Work out the finished part from the listing and answer in its coordinate system (mm). A direction names the side the tool comes from. Coordinates: 2 decimals unless noted, no trailing zeros. Order: outer loops, then holes, each group sorted by start corner. A loop starts at its lowest first (then second) coordinate and runs counter-clockwise, first axis right, second up.
1. The part is cut by section A-A, the plane y = 6. Give the vertices of the cut face in (x, z).
2. The part is cut by section B-B, the plane z = 0. Give the vertices of the cut face in (x, y).
3. Flat-ended cylindrical pins translate along their axes: pin 1 Ø1.2 at (y, z) = (2, -1.5) entering from +X; pin 2 Ø1.2 at (y, z) = (4.5, -2) entering from -X; pin 3 Ø1.2 at (x, y) = (5.5, 5) entering from +Z. Find the tip coordinate at first contact, or state that the pin passes through.
4. The part is cut by section D-D, the plane x = -3.75. Give the vertices of the cut face in (y, z).
5. Find the intervals of material crossed by probe 1 along Z at (x, y) = (-4.02, 7.4); probe 2 along Z at (x, y) = (3, 7.75); probe 3 along X at (y, z) = (4.25, 1.25), in increasing order.
6. Determine the mould class of faces 4 (the flat face through (0, 4, 3.65)), 5 (the flat face through (4.92, 4, 2)), 6 (the cylindrical face through (7.67, 3.85, -0.08)) for opening direction X: +X half, -X half, draft (parallel to the pull), parting line (faces both ways), or undercut.
7. A tool of negligible diameter and unlimited length cuts with its end or side. For faces 1 (the cylindrical face through (-7.067, 7.406, -0.134)), 2 (the flat face through (2, 4, 0.9)), 3 (the cylindrical face through (-7.067, 0.394, 0.134)), from which of +Z, -Z, +X, -X, +Y, -Y can it reach the whole face along a straight path? Write none if from no direction.
8. The part is cut by section C-C, the plane x = 4.5. Give the vertices of the cut face in (y, z), then the cut area to 3 significant figures.
```python
from build123d import *

# Parameters (mm, degrees)
SKETCH1_R           = 2.4
BOSS_EXTRUDE1_DEPTH = 7.8
SKETCH2_R           = 3.05
CUT_EXTRUDE1_DEPTH  = 0.8
SKETCH4_R           = 3.05
CUT_EXTRUDE2_DEPTH  = 0.8


with BuildPart() as part:
    # Sketch1 → Boss-Extrude1 (new body)
    with BuildSketch(Plane(origin=(0, 0, 0), x_dir=(1, 0, 0), z_dir=(0, 1, 0))):
        with BuildLine():
            Line((-4.02, 3.65), (4.02, 3.65))
            ThreePointArc((4.02, 3.65), (7.67, 0), (4.02, -3.65))
            Line((4.02, -3.65), (-4.02, -3.65))
            ThreePointArc((-4.02, -3.65), (-7.67, 0), (-4.02, 3.65))
        make_face()
        with Locations((-4.02, 0)):
            Circle(SKETCH1_R, mode=Mode.SUBTRACT)
        Polygon((3.12, 2.4), (3.12, 0.9), (1.62, 0.9), (1.62, -0.9), (3.12, -0.9), (3.12, -2.4), (4.92, -2.4), (4.92, -0.9), (6.42, -0.9), (6.42, 0.9), (4.92, 0.9), (4.92, 2.4), align=None, mode=Mode.SUBTRACT)
    extrude(amount=BOSS_EXTRUDE1_DEPTH)

    # Sketch2 → Cut-Extrude1 (cut)
    with BuildSketch(Plane(origin=(0, 7.8, 0), x_dir=(1, 0, 0), z_dir=(0, 1, 0))):
        with Locations((-4.02, 0)):
            Circle(SKETCH2_R)
    extrude(amount=-CUT_EXTRUDE1_DEPTH, mode=Mode.SUBTRACT)

    # Sketch4 → Cut-Extrude2 (cut)
    with BuildSketch(Plane.XZ):
        with Locations((-4.02, 0)):
            Circle(SKETCH4_R)
    extrude(amount=-CUT_EXTRUDE2_DEPTH, mode=Mode.SUBTRACT)


solid = part.part
```
Geometry says:
1. outline: (-4.02, -3.65) - (4.02, -3.65) arc R3.65 ccw to (4.02, 3.65) - (-4.02, 3.65) arc R3.65 ccw to start; hole circle Ø4.8 at (-4.02, 0); hole (1.62, -0.9) - (3.12, -0.9) - (3.12, -2.4) - (4.92, -2.4) - (4.92, -0.9) - (6.42, -0.9) - (6.42, 0.9) - (4.92, 0.9) - (4.92, 2.4) - (3.12, 2.4) - (3.12, 0.9) - (1.62, 0.9) - close
2. outline: (-7.67, 0) - (-7.07, 0) - (-7.07, 0.8) - (-6.42, 0.8) - (-6.42, 7) - (-7.07, 7) - (-7.07, 7.8) - (-7.67, 7.8) - close; (-1.62, 0.8) - (-0.97, 0.8) - (-0.97, 0) - (1.62, 0) - (1.62, 7.8) - (-0.97, 7.8) - (-0.97, 7) - (-1.62, 7) - close; (6.42, 0) - (7.67, 0) - (7.67, 7.8) - (6.42, 7.8) - close
3. pin 1: stops at x = 7.56
3. pin 2: stops at x = -7.39
3. pin 3: stops at z = 3.54
4. outline: (0, -3.65) - (7.8, -3.65) - (7.8, -3.04) - (7, -3.04) - (7, -2.38) - (0.8, -2.38) - (0.8, -3.04) - (0, -3.04) - close; (0, 3.04) - (0.8, 3.04) - (0.8, 2.38) - (7, 2.38) - (7, 3.04) - (7.8, 3.04) - (7.8, 3.65) - (0, 3.65) - close
5. probe 1: z = -3.65 to -3.05, 3.05 to 3.65
5. probe 2: z = -3.65 to -0.9, 0.9 to 3.65
5. probe 3: x = -7.45 to -6.07, -1.97 to 3.12, 4.92 to 7.45
6. face 4: draft
6. face 5: undercut
6. face 6: +X half
7. face 1: +Y
7. face 2: +Y, -Y
7. face 3: -Y
8. outline: (0, -3.62) - (7.8, -3.62) - (7.8, -2.4) - (0, -2.4) - close; (0, 2.4) - (7.8, 2.4) - (7.8, 3.62) - (0, 3.62) - close
8. area: 19.0 mm2
